Build history of the part. All positions in model axes, mm. A direction names the side the tool comes from. Give positions to 0.01 mm unless a question says otherwise; leave off trailing zeros. Write each loop counter-clockwise with the first axis right and the second up, starting at its lowest first coordinate (ties: lowest second). Pieces come first, ordered by that corner, then holes. Notation, with made-up numbers: (43.25, -23) -> (96.25, -23) arc R28 ccw to (96.25, 1) -> close; hole circle Ø1 at (48.5, 28.5). An arc over 180 degrees is marked (long way). Put each result on its own line as item: value.
from build123d import *

# Parameters (mm, degrees)
SKETCH1_R           = 49.2
BASE_EXTRUDE_DEPTH  = 3.2
SKETCH5_R           = 3.2
CUT_EXTRUDE2_DEPTH  = 70.652853495
CIRPATTERN1_COUNT   = 4
SKETCH2_R           = 36.5
BOSS_EXTRUDE1_DEPTH = 12.7
SKETCH3_R           = 12.7
BOSS_EXTRUDE2_DEPTH = 12.7
FILLET1_R           = 3.2
SKETCH6_W           = 5.1
SKETCH6_H           = 9.5
BOSS_EXTRUDE3_DEPTH = 47.6
SKETCH4_R           = 7.95
CUT_EXTRUDE1_DEPTH  = 76.227920349
FILLET2_R           = 3.2
CUT_EXTRUDE3_REACH  = 78.92
SKETCH7_R           = 1.6
FILLET3_R           = 1.6


with BuildPart() as part:
    # Sketch1 → Base-Extrude (new body)
    with BuildSketch(Plane.XY):
        Circle(SKETCH1_R)
    extrude(amount=BASE_EXTRUDE_DEPTH)

    # Sketch5 → Cut-Extrude2 (cut, through all)
    with BuildSketch(Plane.XY.offset(3.2)):
        with Locations((31.430896424, 31.430896424)):
            Circle(SKETCH5_R)
    cut_extrude2 = extrude(amount=-CUT_EXTRUDE2_DEPTH, mode=Mode.SUBTRACT)

    # CirPattern1: Cut-Extrude2 ×4 about axis
    cirpattern1_axis = Axis((0, 0, 0), (0, 0, 1))
    for i in range(1, CIRPATTERN1_COUNT):
        add(cut_extrude2.rotate(cirpattern1_axis, i * 360 / CIRPATTERN1_COUNT), mode=Mode.SUBTRACT)

    # Sketch2 → Boss-Extrude1 (add)
    with BuildSketch(Plane.XY.offset(3.2)):
        Circle(SKETCH2_R)
    extrude(amount=BOSS_EXTRUDE1_DEPTH)

    # Sketch3 → Boss-Extrude2 (add)
    with BuildSketch(Plane.XY.offset(15.9)):
        Circle(SKETCH3_R)
    extrude(amount=BOSS_EXTRUDE2_DEPTH)

    # Fillet1
    fillet1_edges = [part.edges().sort_by_distance(p)[0] for p in [
        (-36.5, 0, 3.2),
        (-12.7, 0, 15.9),
    ]]
    fillet(fillet1_edges, radius=FILLET1_R)

    # Sketch6 → Boss-Extrude3 (add)
    with BuildSketch(Plane(origin=(0, 0, 0), x_dir=(1, 0, 0), z_dir=(0, 1, 0))):
        with Locations((0, -7.95)):
            Rectangle(SKETCH6_W, SKETCH6_H)
    extrude(amount=BOSS_EXTRUDE3_DEPTH)

    # Sketch4 → Cut-Extrude1 (cut, through all)
    with BuildSketch(Plane.XY.offset(28.6)):
        Circle(SKETCH4_R)
    extrude(amount=-CUT_EXTRUDE1_DEPTH, mode=Mode.SUBTRACT)

    # Fillet2
    fillet2_edges = [part.edges().sort_by_distance(p)[0] for p in [
        (0, 47.6, 12.7),
    ]]
    fillet(fillet2_edges, radius=FILLET2_R)

    # Sketch7 → Cut-Extrude3 (cut, up to next)
    with BuildSketch(Plane(origin=(2.55, 0, 0), x_dir=(0, 0, -1), z_dir=(1, 0, 0)), mode=Mode.PRIVATE) as cut_extrude3_sk1:
        with Locations((-9.5, 44.4)):
            Circle(SKETCH7_R)
    cut_extrude3_tool1 = extrude(cut_extrude3_sk1.sketch, amount=-CUT_EXTRUDE3_REACH, mode=Mode.PRIVATE) & part.part
    add(cut_extrude3_tool1.solids().sort_by_distance((2.55, 44.4, 9.5))[0], mode=Mode.SUBTRACT)

    # Fillet3
    fillet3_edges = [part.edges().sort_by_distance(p)[0] for p in [
        (2.55, 43.609009945, 3.2),
        (-2.55, 36.410815701, 9.5499997),
        (-2.55, 43.609009945, 3.2),
        (2.55, 36.410815701, 9.5499997),
    ]]
    fillet(fillet3_edges, radius=FILLET3_R)


solid = part.part
1) Slice it at C-C (z = 21.5). Write the cut outline in (x, y).
Filled sheet:
outline: circle Ø25.4 at (0, 0); hole circle Ø15.9 at (0, 0)
2) Slice it at D-D (x = -30). Give the number of separate pieces and of enclosed holes in the cut face, plus the area to 3 significant figures.
Filled sheet:
separate pieces: 3
enclosed holes: 0
area: 748 mm2
3) Pull direction Z, two halves, no side cores. Call faces 4 (the flat face through (10, 1, 0)), 5 (the cylindrical face through (0.04, 44.47, 11.1)), 6 (the flat face through (0, 40, 12.7)), 7 (the cylindrical face through (28.891, 29.484, 1.622)): released by +Z, released by -Z, zero draft, split by the parting line, or undercut.
Filled sheet:
face 4: released by -Z
face 5: undercut
face 6: released by +Z
face 7: zero draft
4) Slice it at A-A (x = 0). Write the cut outline in (y, z).
Filled sheet:
outline: (-49.2, 0) -> (-7.95, 0) -> (-7.95, 28.6) -> (-12.7, 28.6) -> (-12.7, 19.1) arc R3.2 cw to (-15.9, 15.9) -> (-36.5, 15.9) -> (-36.5, 6.4) arc R3.2 cw to (-39.7, 3.2) -> (-49.2, 3.2) -> close; (7.95, 0) -> (49.2, 0) -> (49.2, 3.2) -> (47.6, 3.2) -> (47.6, 9.5) arc R3.2 ccw to (44.4, 12.7) -> (36.5, 12.7) -> (36.5, 15.9) -> (15.9, 15.9) arc R3.2 cw to (12.7, 19.1) -> (12.7, 28.6) -> (7.95, 28.6) -> close; hole circle Ø3.2 at (44.4, 9.5)
5) Pin check, flat tips, straight feed: pin 1 (10 mm diameter, centred on y = -25.5, z = 10, fed in from +X); pin 2 (4 mm diameter, centred on y = 44.4, z = 9.5, fed in from -X); pin 3 (3 mm diameter, centred on x = 2, z = 5, fed in from +Y). Stop position of each tip, or through.
Filled sheet:
pin 1: x = 30.2
pin 2: x = -2.55
pin 3: y = 47.6
6) Tool access for faces 1 (the flat face through (-2.55, 42.7, 8.8)), 2 (the flat face through (0, 47.6, 6)), 3 (the cylindrical face through (-2.75, -12.4, 23.78)): list every direction of +Z, -Z, +X, -X, +Y, -Y with a clear straight run to the whole face (end or side of a thin tool).
Filled sheet:
face 1: +Z, -X, +Y
face 2: +Z, +X, -X, +Y
face 3: +Z
7) Slice it at B-B (y = 0). Write the cut outline in (x, z), plus the area to 3 significant figures.
Filled sheet:
outline: (-49.2, 0) -> (-7.95, 0) -> (-7.95, 28.6) -> (-12.7, 28.6) -> (-12.7, 19.1) arc R3.2 cw to (-15.9, 15.9) -> (-36.5, 15.9) -> (-36.5, 6.4) arc R3.2 cw to (-39.7, 3.2) -> (-49.2, 3.2) -> close; (7.95, 0) -> (49.2, 0) -> (49.2, 3.2) -> (39.7, 3.2) arc R3.2 cw to (36.5, 6.4) -> (36.5, 15.9) -> (15.9, 15.9) arc R3.2 cw to (12.7, 19.1) -> (12.7, 28.6) -> (7.95, 28.6) -> close
area: 1,120 mm2
8) Wall check: L1, parallel to Y at x = 0.45, z = 9.5; L2, parallel to Y at x = -2, z = 9; L3, parallel to Z at x = -11.5, y = 34. Give the ranges that are in metal, low to high.
Filled sheet:
L1: -36.5 to -7.94, 7.94 to 42.8, 46 to 47.6
L2: -36.45 to -7.69, 7.69 to 42.88, 45.92 to 47.6
L3: 0 to 15.9
